Verification items for the finished model (mm, model axes). Face numbers are marked on the shaded views. A direction names the side the tool comes from. Coordinates: 2 decimals unless noted, no trailing zeros. Write each loop counter-clockwise with the first axis right and the second up, starting at its lowest first coordinate (ties: lowest second). Pieces come first, ordered by that corner, then holes. Notation, with made-up numbers: (-28, -20) -> (27, -20) arc R31 ccw to (27, 14) -> close; hole circle Ø9 at (9, 53). An arc over 180 degrees is marked (long way). Answer in a Markdown table with one row per item.
```python
from build123d import *

# Parameters (mm, degrees)
SKETCH1_W           = 40
SKETCH1_H           = 13
BOSS_EXTRUDE1_DEPTH = 6
SKETCH2_W           = 6
SKETCH2_H           = 2
CUT_EXTRUDE1_DEPTH  = 25.596747752
SKETCH3_R           = 0.8
CUT_EXTRUDE2_DEPTH  = 2
SKETCH4_W           = 32
SKETCH4_H           = 7
CUT_EXTRUDE3_DEPTH  = 22.868927729
FILLET1_R           = 4
SKETCH5_R           = 1.5
CUT_EXTRUDE4_DEPTH  = 2
SKETCH6_W           = 6
SKETCH6_H           = 6
BOSS_EXTRUDE2_DEPTH = 20
FILLET3_R           = 6
SKETCH7_R           = 1.5
BOSS_EXTRUDE3_DEPTH = 3
BOSS_EXTRUDE4_START = 3
SKETCH8_R           = 0.8
BOSS_EXTRUDE4_DEPTH = 3


with BuildPart() as part:
    # Sketch1 → Boss-Extrude1 (new body)
    with BuildSketch(Plane(origin=(0, 0, 0), x_dir=(1, 0, 0), z_dir=(0, 1, 0))):
        Rectangle(SKETCH1_W, SKETCH1_H)
    extrude(amount=BOSS_EXTRUDE1_DEPTH)

    # Sketch2 → Cut-Extrude1 (cut, through all)
    with BuildSketch(Plane.XY.offset(6.5)):
        with Locations((-17, 3)):
            Rectangle(SKETCH2_W, SKETCH2_H)
    extrude(amount=-CUT_EXTRUDE1_DEPTH, mode=Mode.SUBTRACT)

    # Sketch3 → Cut-Extrude2 (cut)
    with BuildSketch(Plane(origin=(0, 6, 0), x_dir=(1, 0, 0), z_dir=(0, 1, 0))):
        with Locations(Location((-17, 4, 0), (0, 0, 270))):
            Circle(SKETCH3_R)
        with Locations(Location((-17, -4, 0), (0, 0, 270))):
            Circle(SKETCH3_R)
    extrude(amount=-CUT_EXTRUDE2_DEPTH, mode=Mode.SUBTRACT)

    # Sketch4 → Cut-Extrude3 (cut, through all)
    with BuildSketch(Plane(origin=(0, 6, 0), x_dir=(1, 0, 0), z_dir=(0, 1, 0))):
        with Locations((4, -3)):
            Rectangle(SKETCH4_W, SKETCH4_H)
    extrude(amount=-CUT_EXTRUDE3_DEPTH, mode=Mode.SUBTRACT)

    # Fillet1
    fillet1_edges = [part.edges().sort_by_distance(p)[0] for p in [
        (-12, 3, -0.5),
    ]]
    fillet(fillet1_edges, radius=FILLET1_R)

    # Sketch5 → Cut-Extrude4 (cut)
    with BuildSketch(Plane(origin=(0, 2, 0), x_dir=(1, 0, 0), z_dir=(0, 1, 0))):
        with Locations(Location((-17, 4, 0), (0, 0, 270))):
            Circle(SKETCH5_R)
        with Locations(Location((-17, -4, 0), (0, 0, 270))):
            Circle(SKETCH5_R)
    extrude(amount=-CUT_EXTRUDE4_DEPTH, mode=Mode.SUBTRACT)

    # Sketch6 → Boss-Extrude2 (add)
    with BuildSketch(Plane(origin=(20, 0, 0), x_dir=(0, 0, -1), z_dir=(1, 0, 0))):
        with Locations((3.5, 3)):
            Rectangle(SKETCH6_W, SKETCH6_H)
    extrude(amount=BOSS_EXTRUDE2_DEPTH)

    # Fillet3
    fillet3_edges = [part.edges().sort_by_distance(p)[0] for p in [
        (40, 3, -0.5),
    ]]
    fillet(fillet3_edges, radius=FILLET3_R - 0.0001)  # a hair under: the kernel refuses the full size

    # Sketch7 → Boss-Extrude3 (add)
    with BuildSketch(Plane.XZ):
        with BuildLine():
            Line((-20, -6.5), (40, -6.5))
            ThreePointArc((40, -6.5), (38.242640687, -2.257359313), (34, -0.5))
            Line((34, -0.5), (-8, -0.5))
            ThreePointArc((-8, -0.5), (-10.828427125, 0.671572875), (-12, 3.5))
            Line((-12, 3.5), (-12, 6.5))
            Line((-12, 6.5), (-20, 6.5))
            Line((-20, 6.5), (-20, -6.5))
        make_face()
        with Locations(Location((-17, 4, 0), (0, 0, 90))):
            Circle(SKETCH7_R, mode=Mode.SUBTRACT)
        with Locations(Location((-17, -4, 0), (0, 0, 90))):
            Circle(SKETCH7_R, mode=Mode.SUBTRACT)
    extrude(amount=BOSS_EXTRUDE3_DEPTH)

    # Sketch8 → Boss-Extrude4 (add)
    with BuildSketch(Plane(origin=(0, 6, 0), x_dir=(1, 0, 0), z_dir=(0, 1, 0)).offset(BOSS_EXTRUDE4_START)):
        with BuildLine():
            Line((-8, 0.5), (34, 0.5))
            ThreePointArc((34, 0.5), (38.242640687, 2.257359313), (40, 6.5))
            Line((40, 6.5), (-20, 6.5))
            Line((-20, 6.5), (-20, -6.5))
            Line((-20, -6.5), (-12, -6.5))
            Line((-12, -6.5), (-12, -3.5))
            ThreePointArc((-12, -3.5), (-10.828427125, -0.671572875), (-8, 0.5))
        make_face()
        with Locations(Location((-17, -4, 0), (0, 0, 270))):
            Circle(SKETCH8_R, mode=Mode.SUBTRACT)
        with Locations(Location((-17, 4, 0), (0, 0, 270))):
            Circle(SKETCH8_R, mode=Mode.SUBTRACT)
    extrude(amount=-BOSS_EXTRUDE4_DEPTH)


solid = part.part
```
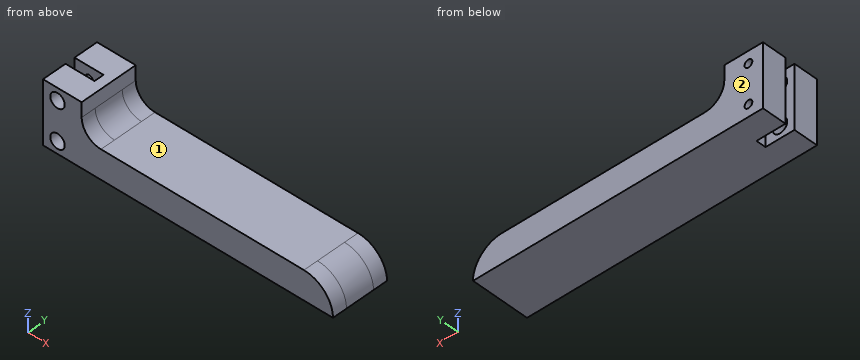
1. Tool access check on the marked faces 1 and 2. Record the directions out of +Z, -Z, +X, -X, +Y, -Y that give a thin tool (end or side, any length) a straight path to the whole face; none if there is none.
Geometry says:
| item | result |
|---|---|
| face 1 | +Z, +X, +Y, -Y |
| face 2 | +Z, -Z, +X, -X, +Y |
2. Section check C-C, the plane z = -4. State how many separate pieces and enclosed holes the cut face has, plus the area to 3 significant figures.
Geometry says:
| item | result |
|---|---|
| separate pieces | 3 |
| enclosed holes | 0 |
| area | 678 mm^2 |
3. Section check A-A, the plane x = -17. Record the boundary of the cut face in (y, z), plus the area to 3 significant figures.
Geometry says:
| item | result |
|---|---|
| outline | (-3, -6.5) -> (2, -6.5) -> (2, -5.5) -> (-3, -5.5) -> close; (-3, -2.5) -> (2, -2.5) -> (2, 2.5) -> (-3, 2.5) -> close; (-3, 5.5) -> (2, 5.5) -> (2, 6.5) -> (-3, 6.5) -> close; (4, -6.5) -> (9, -6.5) -> (9, -4.8) -> (4, -4.8) -> close; (4, -3.2) -> (9, -3.2) -> (9, 3.2) -> (4, 3.2) -> close; (4, 4.8) -> (9, 4.8) -> (9, 6.5) -> (4, 6.5) -> close |
| area | 84.0 mm^2 |
4. Thickness scan on line 1 (Z direction, x = -17, y = -0.8); line 2 (X direction, y = 7.75, z = 4); line 3 (Z direction, x = 15, y = -0.5). Record the ranges inside material, lowest first. Write a range as from..to.
Geometry says:
| item | result |
|---|---|
| line 1 | -6.5..-5.5, -2.5..2.5, 5.5..6.5 |
| line 2 | -20..-17.8, -16.2..-12 |
| line 3 | -6.5..-0.5 |
5. Depth check by flat-ended pin: P1, Ø3, axis at x = 16, y = 7.5, coming from the +Z side; P2, Ø3, axis at y = 3.5, z = 2.5, coming from the +X side; P3, Ø0.9, axis at y = 1, z = 4.5, coming from the +X side. Enter the tip coordinate at first touch or a pass-through.
Geometry says:
| item | result |
|---|---|
| P1 | z = -0.5 |
| P2 | x = -11.12 |
| P3 | x = -12 |
6. Section check D-D, the plane z = 1.25. Record the boundary of the cut face in (x, y), plus the area to 3 significant figures.
Geometry says:
| item | result |
|---|---|
| outline | (-20, -3) -> (-11.31, -3) -> (-11.31, 9) -> (-20, 9) -> (-20, 4) -> (-14, 4) -> (-14, 2) -> (-20, 2) -> close |
| area | 92.3 mm^2 |
